Geometry: final body of the model. Coordinates: model frame, mm. Round coordinates to 2 decimals unless told otherwise and drop trailing zeros. Write each loop counter-clockwise with the first axis right and the second up, starting at its lowest first coordinate (ties: lowest second). Pieces come first, ordered by that corner, then holes. Notation, with made-up numbers: M 79.5,58 L 103.5,58 A20 ccw 103.5,96 Z; hole C 38,7.25 d8. An arc over 180 degrees is marked long. Use one line per item in the form item = value. Start each with the question number.
from build123d import *

# Parameters (mm, degrees)
BOSS_EXTRUDE1_DEPTH      = 50
BOSS_EXTRUDE1_DEPTH_BACK = 50
FILLET1_R                = 30
BOSS_EXTRUDE2_DEPTH      = 4
FILLET4_R                = 20


with BuildPart() as part:
    # Sketch1 → Boss-Extrude1 (new, two sides: drawn at the far end of the back side and taken through both)
    with BuildSketch(Plane(origin=(0, 0, 0), x_dir=(0, 0, -1), z_dir=(1, 0, 0)).offset(-BOSS_EXTRUDE1_DEPTH_BACK)):
        with BuildLine():
            Line((67.5, -28.571428571), (40, 50))
            Line((40, 50), (-25.000000097, 50))
            ThreePointArc((-25.000000097, 50), (-75, -6.7e-08), (-24.999999963, -50))
            Line((-24.999999963, -50), (67.5, -50))
            Line((67.5, -50), (67.5, -28.571428571))
        make_face()
    extrude(amount=BOSS_EXTRUDE1_DEPTH + BOSS_EXTRUDE1_DEPTH_BACK)

    # Fillet1
    fillet1_edges = [part.edges().sort_by_distance(p)[0] for p in [
        (0, 50, -40),
    ]]
    fillet(fillet1_edges, radius=FILLET1_R)

    # Sketch6 → Boss-Extrude2 (add)
    with BuildSketch(Plane(origin=(50, 0, 0), x_dir=(0, 0, -1), z_dir=(1, 0, 0))):
        with BuildLine():
            ThreePointArc((-1.291867628, -35), (0.59665296, -32.49963092), (1.075777558, -29.403052943))
            Line((1.075777558, -29.403052943), (1.837060492, -15))
            ThreePointArc((1.837060492, -15), (-12.80850841, -6.144567228), (-13.846677423, -23.22770462))
            Line((-13.846677423, -23.22770462), (-11.38303259, -27.92393056))
            ThreePointArc((-11.38303259, -27.92393056), (-11.474733065, -31.785574712), (-9.332730592, -35))
            Line((-9.332730592, -35), (-1.291867628, -35))
        make_face()
    boss_extrude2 = extrude(amount=BOSS_EXTRUDE2_DEPTH)

    # Mirror2: Boss-Extrude2 across plane
    add(boss_extrude2.mirror(Plane(origin=(0, 0, 0), x_dir=(0, 0, 1), z_dir=(1, 0, 0))))

    # Fillet4
    fillet4_edges = [part.edges().sort_by_distance(p)[0] for p in [
        (0, -50, -67.5),
    ]]
    fillet(fillet4_edges, radius=FILLET4_R)


solid = part.part
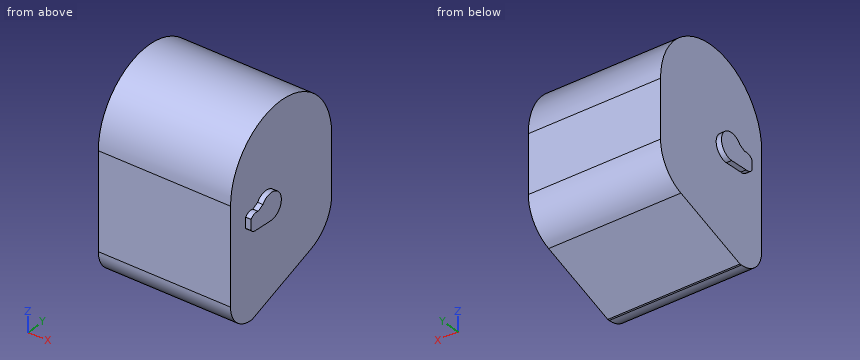
1. Contact query for flat-ended pins moving along their axis: pin 1 (1.5 mm diameter, centred on x = -2.5, y = -1, fed in from -Z); pin 2 (10 mm diameter, centred on y = -12.5, z = -8.5, fed in from -X); pin 3 (10 mm diameter, centred on x = -6, z = -34.5, fed in from +Y). Output: stop coordinate, or through.
2. Ray query, probe 1 along X at (y, z) = (16.5, -33.5); probe 2 along Z at (x, y) = (4, -4); probe 3 along Y at (x, z) = (45.5, 57.5). Return the intervals inside material, ascending.
3. Section query C-C (y = 0). Return loops of the section in (x, z).
4. Section query A-A (x = 1). Return loops of the section in (y, z), then the cut area to 3 significant figures.
5. Section query B-B (z = -16). Return loops of the section in (x, y).
Checks:
q1.pin_1 = -58.11
q1.pin_2 = -50
q1.pin_3 = 47.99
q2.probe_1 = -50 to 50
q2.probe_2 = -58.9 to 74.84
q2.probe_3 = -38 to 38
q3.outline = M -50,-57.5 L 50,-57.5 L 50,75 L -50,75 Z
q4.outline = M -50,-47.5 A20 ccw -30,-67.5 L -28.57,-67.5 L 29.91,-47.03 A30 ccw 50,-18.72 L 50,25 A50 ccw -50,25 Z
q4.area = 11,900 mm^2
q5.outline = M -50,-50 L 50,-50 L 50,50 L -50,50 Z
